Part model, mm, in its own coordinate system. A direction names the side the tool comes from. Round coordinates to 2 decimals unless told otherwise and drop trailing zeros. Loops run counter-clockwise (first coordinate to the right, second up) from the corner with the lowest first, then second, coordinate; pieces in that order, holes last.
(1) Tool access for faces 1 (the face through (-26.49, 14.48, 5.04)), 2 (the face through (-24.16, 13.666, 4.93)), 3 (the face through (-26.566, 11, 5)): list every direction of +Z, -Z, +X, -X, +Y, -Y with a clear straight run to the whole face (end or side of a thin tool).
(2) Cut at C-C on z = 8.75. List the corners of the cut face in (x, y).
(3) Probe probe 1 along Y at (x, z) = (-22, 1.5); probe 2 along X at (y, z) = (11, 7.25); probe 3 along Y at (x, z) = (-31.5, 4.5). List the from-to ranges inside material, lowest first.
(4) Cut at A-A on x = -16. List the corners of the cut face in (y, z).
(5) Mould opens along Y. For faces 4 (the face through (-9.566, 11, 5)), 5 (the face through (-33.566, 13, 5)), 6 (the face through (-16, 6.807, 5)), 7 (the face through (-7.115, 14.649, 2.708)) say: +Y half, -Y half, draft (parallel to the pull), parting line (faces both ways), or undercut.
(6) Flat gauge pins, fed straight in: pin 1 (1.5 mm diameter, centred on y = 16, z = 3.5, fed in from +X); pin 2 (2 mm diameter, centred on x = -4, z = 7.5, fed in from -Y); pin 3 (5.5 mm diameter, centred on x = -4.5, z = 3, fed in from +Y); pin 4 (2.5 mm diameter, centred on x = -4.57, z = 5, fed in from -Y). Where does each tip first touch, or does it go through?
(7) Cut at B-B on y = 11.25. List the corners of the cut face in (x, z), then the cut area to 3 significant figures.
(8) Cut at D-D on y = 13.25. List the corners of the cut face in (x, z), then the cut area to 3 significant figures.
from build123d import *

# Parameters (mm, degrees)
F1_DEPTH = 10
F2_R     = 1.55
F3_DEPTH = 5
F4_R     = 3.075
F5_DEPTH = 5
F6_R     = 3.075
F7_DEPTH = 5


# Not quite as in the source:
# - a feature names something its author has since deleted; it is built from what else it names


with BuildPart() as f1:
    # F0 (on Top) → F1 (new body)
    with BuildSketch(Plane.XY):
        with BuildLine():
            Line((-1.5664058328, 14.3066409416), (-5.9960383158, 14.3066409416))
            ThreePointArc((-5.9960383158, 14.3066409416), (-6.9397541669, 14.5432917441), (-7.6601389045, 15.1972405492))
            Line((-7.6601389045, 15.1972405492), (-8.3242394931, 16.1933914322))
            ThreePointArc((-8.3242394931, 16.1933914322), (-8.8670406285, 16.7780954993), (-9.5664058328, 17.1620228746))
            ThreePointArc((-9.5664058328, 17.1620228746), (-9.9791916365, 17.2702211446), (-10.404365229, 17.3066409416))
            Line((-10.404365229, 17.3066409416), (-23.2284464365, 17.3066409416))
            ThreePointArc((-23.2284464365, 17.3066409416), (-24.4080912504, 17.0108274386), (-25.3085721724, 16.1933914322))
            Line((-25.3085721724, 16.1933914322), (-25.9726727611, 15.1972405492))
            ThreePointArc((-25.9726727611, 15.1972405492), (-26.6930574987, 14.5432917441), (-27.6367733497, 14.3066409416))
            Line((-27.6367733497, 14.3066409416), (-32.5664058328, 14.3066409416))
            Line((-32.5664058328, 14.3066409416), (-33.5664058328, 14.3066409416))
            Line((-33.5664058328, 14.3066409416), (-33.5664058328, 12.3066409416))
            Line((-33.5664058328, 12.3066409416), (-32.5664058328, 12.3066409416))
            Line((-32.5664058328, 12.3066409416), (-26.5664058328, 12.3066409416))
            Line((-26.5664058328, 12.3066409416), (-26.5664058328, 9.3240286596))
            ThreePointArc((-26.5664058328, 9.3240286596), (-26.3794394083, 8.3840849704), (-25.8470040783, 7.5872391872))
            Line((-25.8470040783, 7.5872391872), (-23.8748829035, 5.6151180124))
            ThreePointArc((-23.8748829035, 5.6151180124), (-22.979372793, 5.0167572865), (-21.9230465945, 4.8066409416))
            Line((-21.9230465945, 4.8066409416), (-9.2356068064, 4.8066409416))
            ThreePointArc((-9.2356068064, 4.8066409416), (-8.0553034788, 5.2955385877), (-7.5664058328, 6.4758419153))
            Line((-7.5664058328, 6.4758419153), (-7.5664058328, 12.3066409416))
            Line((-7.5664058328, 12.3066409416), (-1.5664058328, 12.3066409416))
            Line((-1.5664058328, 12.3066409416), (-0.5664058328, 12.3066409416))
            Line((-0.5664058328, 12.3066409416), (-0.5664058328, 14.3066409416))
            Line((-0.5664058328, 14.3066409416), (-1.5664058328, 14.3066409416))
        make_face()
        Polygon((-9.5664058328, 14.8066409416), (-9.5664058328, 6.8066409416), (-22.5664058328, 6.8066409416), (-25.0664058328, 9.0566409416), (-25.0664058328, 10.8066409416), (-25.0664058328, 12.5566409416), (-23.2284464365, 14.8066409416), (-22.5664058328, 14.8066409416), align=None, mode=Mode.SUBTRACT)
    extrude(amount=F1_DEPTH)

    # F2 (on face) → F3 (cut)
    with BuildSketch(Plane.XZ.offset(-12.3066409416)):
        with Locations((-29.5664058328, 5)):
            Circle(F2_R)
        with Locations((-4.5664058328, 5)):
            Circle(F2_R)
    extrude(amount=-F3_DEPTH, mode=Mode.SUBTRACT)

    # F4 (on face) → F5 (cut)
    with BuildSketch(Plane(origin=(0, 14.3066409416, 0), x_dir=(-1, 0, 0), z_dir=(0, 1, 0))):
        with Locations((29.5664058328, 5)):
            Circle(F4_R)
    extrude(amount=F5_DEPTH, mode=Mode.SUBTRACT)

    # F6 (on face) → F7 (cut)
    with BuildSketch(Plane(origin=(0, 14.3066409416, 0), x_dir=(-1, 0, 0), z_dir=(0, 1, 0))):
        with Locations((4.5664058328, 5)):
            Circle(F6_R)
    extrude(amount=F7_DEPTH, mode=Mode.SUBTRACT)


solid = f1.part
Final values:
1. face 1: -X, +Y
1. face 2: +Z, -Z
1. face 3: +Z, -Z, -X, -Y
2. outline: (-33.57, 12.31) - (-26.57, 12.31) - (-26.57, 9.32) arc R2.46 ccw to (-25.85, 7.59) - (-23.87, 5.62) arc R2.76 ccw to (-21.92, 4.81) - (-9.24, 4.81) arc R1.67 ccw to (-7.57, 6.48) - (-7.57, 12.31) - (-0.57, 12.31) - (-0.57, 14.31) - (-6, 14.31) arc R2 cw to (-7.66, 15.2) - (-8.32, 16.19) arc R2.5 ccw to (-10.4, 17.31) - (-23.23, 17.31) arc R2.5 ccw to (-25.31, 16.19) - (-25.97, 15.2) arc R2 cw to (-27.64, 14.31) - (-33.57, 14.31) - close; hole (-25.07, 9.06) - (-22.57, 6.81) - (-9.57, 6.81) - (-9.57, 14.81) - (-23.23, 14.81) - (-25.07, 12.56) - close
3. probe 1: y = 4.81 to 6.81, 14.81 to 17.31
3. probe 2: x = -26.57 to -25.07, -9.57 to -7.57
3. probe 3: y = 12.31 to 14.31
4. outline: (4.81, 0) - (6.81, 0) - (6.81, 10) - (4.81, 10) - close; (14.81, 0) - (17.31, 0) - (17.31, 10) - (14.81, 10) - close
5. face 4: undercut
5. face 5: draft
5. face 6: undercut
5. face 7: +Y half
6. pin 1: stops at x = -7.7
6. pin 2: stops at y = 12.31
6. pin 3: stops at y = 14.75
6. pin 4: passes through
7. outline: (-26.57, 0) - (-25.07, 0) - (-25.07, 10) - (-26.57, 10) - close; (-9.57, 0) - (-7.57, 0) - (-7.57, 10) - (-9.57, 10) - close
7. area: 35.0 mm2
8. outline: (-33.57, 0) - (-24.5, 0) - (-24.5, 10) - (-33.57, 10) - close; (-9.57, 0) - (-0.57, 0) - (-0.57, 10) - (-9.57, 10) - close; hole circle Ø3.1 at (-29.57, 5); hole circle Ø3.1 at (-4.57, 5)
8. area: 166 mm2
